Check sheet for the drawn part. Datum: minimum x, y, z corner. Units: mm. A direction names the side the tool comes from. Round coordinates to 2 decimals unless told otherwise and drop trailing zeros. Write each loop counter-clockwise with the first axis right and the second up, starting at its lowest first coordinate (ties: lowest second). Pieces come first, ordered by that corner, then holes. Notation, with made-up numbers: (65, -0.75) - (88, -0.75) arc R24 cw to (88, 34.25) - close; hole circle Ø9 at (79, 28). An arc over 180 degrees is marked (long way). Answer as a JSON object with one key per item and string values.
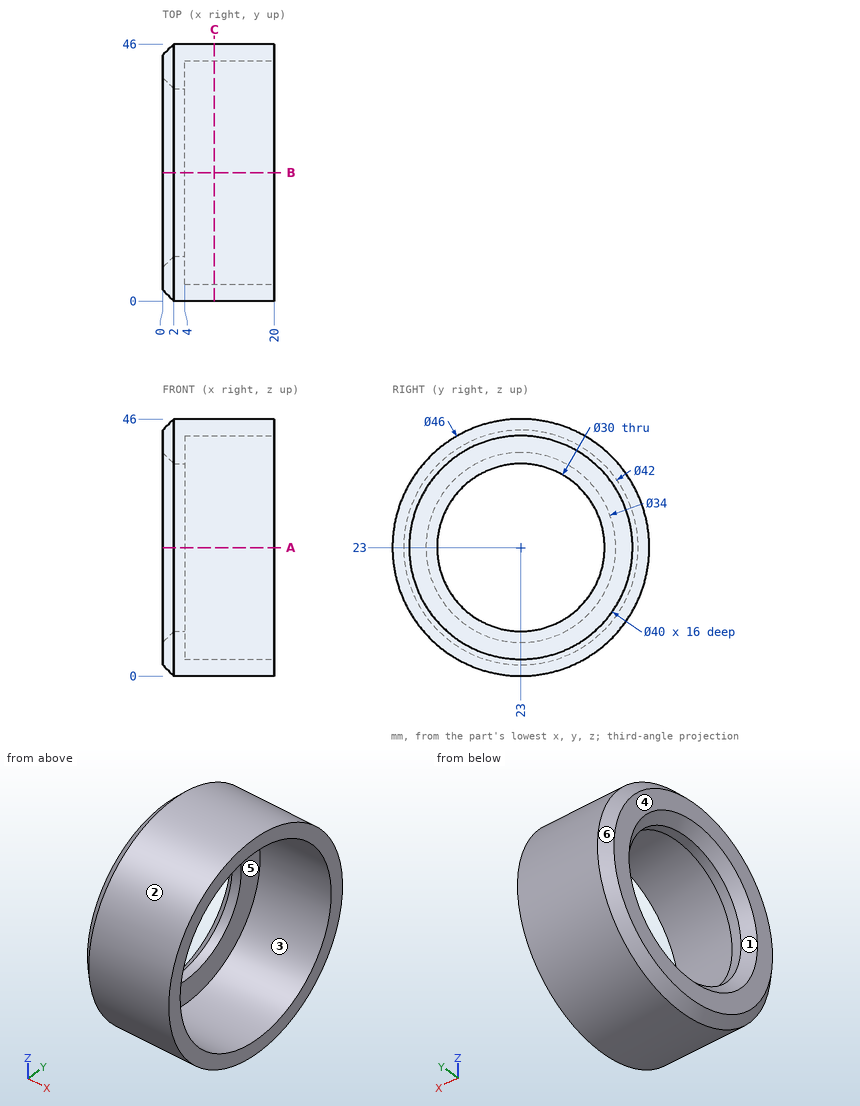
1. Cross-section at A-A (z = 23). Record the boundary of the cut face in (x, y), plus the area to 3 significant figures.
Completed:
{"outline": "(0, 2) - (2, 0) - (20, 0) - (20, 3) - (4, 3) - (4, 8) - (2, 8) - (0, 6) - close; (0, 40) - (2, 38) - (4, 38) - (4, 43) - (20, 43) - (20, 46) - (2, 46) - (0, 44) - close", "area": "152 mm^2"}
2. Access from +Z, -Z, +X, -X, +Y, -Y to the whole of each face (thin tool, end or side, straight path). Record for the marked faces 5 and 6.
Completed:
{"face 5": "+X", "face 6": "-X"}
3. Go/stop test with flat-tipped pins: pin 1 (1 mm diameter, centred on y = 39, z = 22.5, fed in from -X); pin 2 (6 mm diameter, centred on x = 17, y = 36.5, fed in from -Z); pin 3 (5 mm diameter, centred on x = 10, z = 22, fed in from -Y). Record where each tip stops, or that it passes through.
Completed:
{"pin 1": "stops at x = 0.49", "pin 2": "stops at z = 2.54", "pin 3": "stops at y = 0"}
4. Mould release check, pull along Y, two halves, no side actions. Record for the marked faces 1, 2, 3 and 4: released by +Y, released by -Y, zero draft, split by the parting line, or undercut.
Completed:
{"face 1": "undercut", "face 2": "split by the parting line", "face 3": "undercut", "face 4": "zero draft"}
5. Material ranges on probe 1 along Z at (x, y) = (13.75, 23); probe 2 along Y at (x, z) = (3.4, 23), recorded low to high. Write a range as from..to.
Completed:
{"probe 1": "z = 0..3, 43..46", "probe 2": "y = 0..8, 38..46"}
6. Cross-section at C-C (x = 9.25). Record the boundary of the cut face in (y, z), plus the area to 3 significant figures.
Completed:
{"outline": "circle Ø46 at (23, 23); hole circle Ø40 at (23, 23)", "area": "405 mm^2"}
